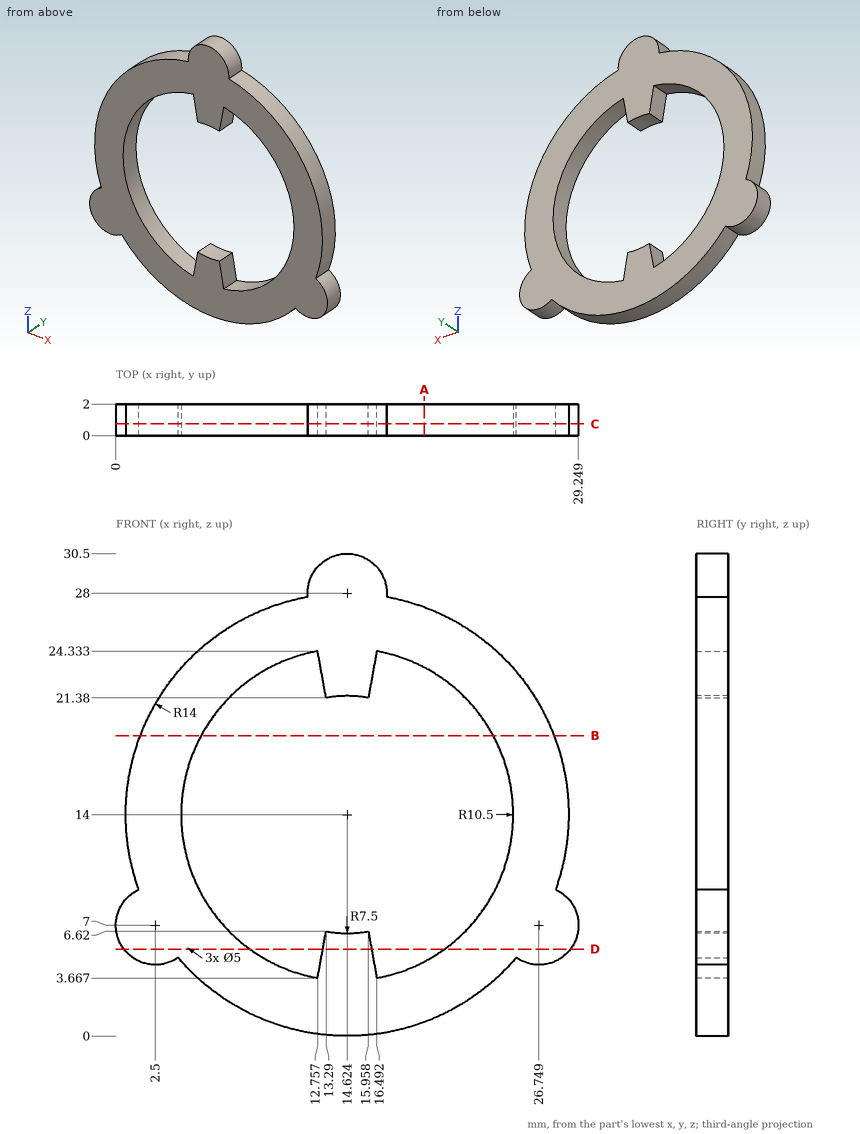
Drawing for the job (mm, zero at the part's lowest x, y, z). Give positions to 0.01 mm unless a question says otherwise; leave off trailing zeros. Order: outer loops, then holes, each group sorted by start corner. A loop starts at its lowest first (then second) coordinate and runs counter-clockwise, first axis right, second up. Notation, with made-up numbers: M 11,53.5 L 47,53.5 A27 ccw 47,84.5 Z; hole C 22,39 d6. An arc over 180 degrees is marked long. Put each result on its own line as item: value. Start each with the question number.
(1) Saw through at C-C, the plane y = 0.75. Write the cut outline in (x, z) (1 decimal), then the cut area to 3 significant figures.
(2) Saw through at B-B, the plane z = 19. Write the cut outline in (x, y), then the cut area to 3 significant figures.
(3) Saw through at D-D, the plane z = 5.5. Write the cut outline in (x, y).
(4) Saw through at A-A, the plane x = 19.5. Write the cut outline in (y, z), then the cut area to 3 significant figures.
(5) Drill centre lines: line 1 along X through (y, z) = (0.65, 22) (1 decimal); line 2 along X through (y, z) = (1, 6) (1 decimal); line 3 along Z through (x, y) = (19.25, 1.85) (1 decimal). Where is each one in solid material? Low to high.
Check result:
1. outline: M 1.4,9.3 A2.5 ccw long 3.9,5 A14 ccw 25.3,5 A2.5 ccw long 27.8,9.3 A14 ccw 17.1,27.8 A2.5 ccw long 12.1,27.8 A14 ccw Z; hole M 12.8,3.7 L 13.3,6.6 A7.5 ccw 16,6.6 L 16.5,3.7 A10.5 ccw 16.5,24.3 L 16,21.4 A7.5 ccw 13.3,21.4 L 12.8,24.3 A10.5 ccw Z
1. area: 319 mm2
2. outline: M 1.55,0 L 5.39,0 L 5.39,2 L 1.55,2 Z; M 23.86,0 L 27.7,0 L 27.7,2 L 23.86,2 Z
2. area: 15.4 mm2
3. outline: M 0.5,0 L 8.46,0 L 8.46,2 L 0.5,2 Z; M 13.09,0 L 16.16,0 L 16.16,2 L 13.09,2 Z; M 20.79,0 L 28.75,0 L 28.75,2 L 20.79,2 Z
4. outline: M 0,0.88 L 2,0.88 L 2,4.7 L 0,4.7 Z; M 0,23.3 L 2,23.3 L 2,27.12 L 0,27.12 Z
4. area: 15.3 mm2
5. line 1: x = 3.1 to 7.8, 13.2 to 16.1, 21.4 to 26.1
5. line 2: x = 0.2 to 7.8, 13.2 to 16.1, 21.4 to 29
5. line 3: z = 0.8 to 4.6, 23.4 to 27.2
